Part model, mm, in its own coordinate system. A direction names the side the tool comes from. Round coordinates to 2 decimals unless told otherwise and drop trailing zeros. Loops run counter-clockwise (first coordinate to the right, second up) from the corner with the lowest first, then second, coordinate; pieces in that order, holes last. Notation, with made-up numbers: M 1,-31.5 L 60,-31.5 A20 ccw 60,-19.5 Z; hole C -27.75,64 d1. An arc over 180 degrees is marked long. Write each question's results on one line, items separated by ' | '.
from build123d import *

# Parameters (mm, degrees)
F0_W     = 8
F0_H     = 8
F0_W_2   = 7
F0_H_2   = 7
F1_DEPTH = 1
F3_DEPTH = 2.5
F4_R     = 1
F5_DEPTH = 2.501
F6_SIZE  = 1


with BuildPart() as f1:
    # F0 (on Top) → F1 (new body)
    with BuildSketch(Plane.XY):
        Rectangle(F0_W, F0_H)
        with Locations((-7.5, 0)):
            Rectangle(F0_W_2, F0_H)
        with Locations((0, 7.5)):
            Rectangle(F0_W, F0_H_2)
        with Locations((0, -7.5)):
            Rectangle(F0_W, F0_H_2)
        with Locations((7.5, 0)):
            Rectangle(F0_W_2, F0_H)
    extrude(amount=F1_DEPTH)

    # F2 (on Top) → F3 (join)
    with BuildSketch(Plane.XY):
        with BuildLine():
            ThreePointArc((2.036100952, 11), (4.945464062, 19.7962570079), (0, 27.630854398))
            ThreePointArc((0, 27.630854398), (-5.0783073922, 19.8178102809), (-2.0651551895, 11))
            Line((-2.0651551895, 11), (2.036100952, 11))
        make_face()
        with BuildLine():
            Line((-11, -1.9892101258), (-11, 2.4604453852))
            ThreePointArc((-11, 2.4604453852), (-19.4622945933, 4.4658207731), (-26.9247610122, 0))
            ThreePointArc((-26.9247610122, 0), (-19.3807111434, -4.3435802853), (-11, -1.9892101258))
        make_face()
        with BuildLine():
            Line((2.6823603006, -11), (-2.3196401929, -11))
            ThreePointArc((-2.3196401929, -11), (-4.574812793, -19.1721128853), (0, -26.3093616813))
            ThreePointArc((0, -26.3093616813), (4.36279709, -19.1840997342), (2.6823603006, -11))
        make_face()
        with BuildLine():
            ThreePointArc((11, -1.9892101258), (19.9655151881, -4.5182315612), (28.1118024141, 0))
            ThreePointArc((28.1118024141, 0), (20.0578865698, 4.7214094483), (11, 2.4604453852))
            Line((11, 2.4604453852), (11, -1.9892101258))
        make_face()
    extrude(amount=F3_DEPTH)

    # F4 (on face) → F5 (cut, through all)
    with BuildSketch(Plane(origin=(0, 0, 0), x_dir=(1, 0, 0), z_dir=(0, 0, -1))):
        with Locations((0, 14)):
            Circle(F4_R)
        with Locations((-14, 0)):
            Circle(F4_R)
        with Locations((0, -14)):
            Circle(F4_R)
        with Locations((14, 0)):
            Circle(F4_R)
    extrude(amount=-F5_DEPTH, mode=Mode.SUBTRACT)

    # F6
    f6_edges = [f1.edges().sort_by_distance(p)[0] for p in [
        (-5.078307, 19.81781, 2.5),
        (4.945464, 19.796257, 2.5),
        (20.057887, 4.721409, 2.5),
        (4.362797, -19.1841, 2.5),
        (19.965515, -4.518232, 2.5),
        (-4.574813, -19.172113, 2.5),
        (-19.462295, 4.465821, 2.5),
        (-19.380711, -4.34358, 2.5),
    ]]
    chamfer(f6_edges, length=F6_SIZE)


solid = f1.part
Item 1: Band-saw the part on A-A on z = 0.5. Give the cut face in (x, y), and give its area (3 significant figures).
Filled sheet:
outline: M -26.92,0 A11.23 ccw -11,-1.99 L -11,-4 L -4,-4 L -4,-11 L -2.32,-11 A10.4 ccw 0,-26.31 A11.38 ccw 2.68,-11 L 4,-11 L 4,-4 L 11,-4 L 11,-1.99 A12.23 ccw 28.11,0 A12.36 ccw 11,2.46 L 11,4 L 4,4 L 4,11 L 2.04,11 A10.85 ccw 0,27.63 A10.65 ccw -2.07,11 L -4,11 L -4,4 L -11,4 L -11,2.46 A11.55 ccw Z; hole C -14,0 d2; hole C 0,-14 d2; hole C 0,14 d2; hole C 14,0 d2 | area: 743 mm^2
Item 2: Two-plate mould, pull along X, no slides. Class faces 3 (the conical face through (-4.286, 19.313, 2.34)), 4 (the flat face through (-11, 0, 2)), 5 (the conical face through (3.57, -18.82, 2.34)), 6 (the flat face through (19, 0, 2.5)): +X half, -X half, draft (parallel to the pull), parting line (faces both ways), or undercut.
Filled sheet:
face 3: -X half | face 4: undercut | face 5: +X half | face 6: draft
Item 3: Wall check: L1, parallel to Y at x = -14, z = 0.8; L2, parallel to X at y = 0, z = 1.65; L3, parallel to X at y = 0, z = 1.9. Give the ranges that are in metal, low to high.
Filled sheet:
L1: -3.7 to -1, 1 to 3.99 | L2: -26.74 to -15, -13 to -11, 11 to 13, 15 to 27.92 | L3: -26.42 to -15, -13 to -11, 11 to 13, 15 to 27.59
Item 4: Band-saw the part on B-B on x = -3. Count the separate pieces of the cut face and the enclosed holes in it, and give its area (3 significant figures).
Filled sheet:
separate pieces: 3 | enclosed holes: 0 | area: 78.8 mm^2
Item 5: Which spindle directions (+Z, -Z, +X, -X, +Y, -Y) get a long thin tool onto all of the face, cutting with end or side? Do faces 1 (the flat face through (11, 0, 2)), 2 (the conical face through (4.17, 19.06, 2.34)). Say none if no direction does.
Filled sheet:
face 1: +Z, +Y, -Y | face 2: +Z, +X
Item 6: Drop flat-ended pins along their axis: P1, Ø0.5, axis at y = 1, z = 2, coming from the +X side; P2, Ø0.8, axis at y = 8.5, z = 0.5, coming from the +X side; P3, Ø0.8, axis at x = 6.5, z = 0.5, coming from the -Y side. Give the stop position or say it passes through.
Filled sheet:
P1: x = 26.99 | P2: x = 4 | P3: y = -4
